The listing builds one solid part. Answer for the finished solid, in the listing's coordinates (mm). A direction names the side the tool comes from. Give positions to 0.01 mm unless a question says otherwise; leave off trailing zeros. Order: outer loops, then holes, each group sorted by start corner. A loop starts at its lowest first (then second) coordinate and runs counter-clockwise, first axis right, second up.
```python
from build123d import *

# Parameters (mm, degrees)
SKETCH1_R           = 1.8415
BOSS_EXTRUDE1_DEPTH = 3.81
CUT_EXTRUDE2_DEPTH  = 3.81
SKETCH2_R           = 3.4925
BOSS_EXTRUDE2_DEPTH = 31.75
SKETCH4_R           = 5.001975
SKETCH4_R_2         = 1.8415
SKETCH4_R_3         = 5.08
BOSS_EXTRUDE3_DEPTH = 6.35
SKETCH6_R           = 1.778
CUT_EXTRUDE3_DEPTH  = 5.08


with BuildPart() as part:
    # Sketch1 → Boss-Extrude1 (new body)
    with BuildSketch(Plane(origin=(0, 0, 0), x_dir=(1, 0, 0), z_dir=(0, 1, 0))):
        with BuildLine():
            Line((35.013825, 0), (38.50005, -3.486225))
            Line((38.50005, -3.486225), (41.802802741, -3.486225))
            ThreePointArc((41.802802741, -3.486225), (50.162319809, -2.012011059), (45.49775, 5.08))
            Line((45.49775, 5.08), (38.50005, 5.08))
            Line((38.50005, 5.08), (38.50005, 29.9974))
            Line((38.50005, 29.9974), (8.48995, 29.9974))
            Line((8.48995, 29.9974), (8.48995, 34.7599))
            ThreePointArc((8.48995, 34.7599), (3.40995, 39.8399), (-1.67005, 34.7599))
            Line((-1.67005, 34.7599), (-1.67005, 29.9974))
            Line((-1.67005, 29.9974), (-38.50005, 29.9974))
            Line((-38.50005, 29.9974), (-38.50005, 5.001975))
            ThreePointArc((-38.50005, 5.001975), (-42.036980442, -3.536930442), (-33.498075, 0))
            Line((-33.498075, 0), (35.013825, 0))
        make_face()
        with Locations((3.40995, 34.7599)):
            Circle(SKETCH1_R, mode=Mode.SUBTRACT)
        with Locations((45.49775, 0)):
            Circle(SKETCH1_R, mode=Mode.SUBTRACT)
        with Locations((-38.50005, 0)):
            Circle(SKETCH1_R, mode=Mode.SUBTRACT)
    extrude(amount=BOSS_EXTRUDE1_DEPTH)

    # Sketch3 → Cut-Extrude2 (cut)
    with BuildSketch(Plane(origin=(0, 0, 0), x_dir=(1, 0, 0), z_dir=(0, 1, 0))):
        with BuildLine():
            Line((-38.50005, 8.176975), (-38.50005, 29.9974))
            Line((-38.50005, 29.9974), (-4.84505, 29.9974))
            ThreePointArc((-4.84505, 29.9974), (-17.79061216, 13.099833084), (-38.50005, 8.176975))
        make_face()
    extrude(amount=CUT_EXTRUDE2_DEPTH, mode=Mode.SUBTRACT)

    # Sketch2 → Boss-Extrude2 (add)
    with BuildSketch(Plane(origin=(0, 0, 0), x_dir=(1, 0, 0), z_dir=(0, 1, 0))):
        with Locations((-15.55115, 14.9963886)):
            Circle(SKETCH2_R)
        with Locations((22.54885, 14.9963886)):
            Circle(SKETCH2_R)
    extrude(amount=BOSS_EXTRUDE2_DEPTH)

    # Sketch4 → Boss-Extrude3 (add)
    with BuildSketch(Plane.XZ):
        with Locations((-38.50005, 0)):
            Circle(SKETCH4_R)
        with Locations((-38.50005, 0)):
            Circle(SKETCH4_R_2, mode=Mode.SUBTRACT)
        with Locations((45.49775, 0)):
            Circle(SKETCH4_R_3)
        with Locations((45.49775, 0)):
            Circle(SKETCH4_R_2, mode=Mode.SUBTRACT)
        with Locations((3.40995, -34.7599)):
            Circle(SKETCH4_R_3)
        with Locations((3.40995, -34.7599)):
            Circle(SKETCH4_R_2, mode=Mode.SUBTRACT)
    extrude(amount=BOSS_EXTRUDE3_DEPTH)

    # Sketch6 → Cut-Extrude3 (cut)
    with BuildSketch(Plane(origin=(0, 31.75, 0), x_dir=(1, 0, 0), z_dir=(0, 1, 0))):
        with Locations((-15.55115, 14.9963886)):
            Circle(SKETCH6_R)
    extrude(amount=-CUT_EXTRUDE3_DEPTH, mode=Mode.SUBTRACT)


solid = part.part
```
1) For a pull along X with two mould halves and no side action, classify faces 4 (the cylindrical face through (-18.125, 15.653, -17.357)), 5 (the cylindrical face through (2.31, -2.33, -39.72)), 6 (the flat face through (38.5, 2, -17)), 7 (the cylindrical face through (-40.34, -1.2, 0.08)) as +X half, -X half, draft (parallel to the pull), parting line (faces both ways), or undercut.
Geometry says:
face 4: undercut
face 5: parting line
face 6: +X half
face 7: undercut
2) Given P1, Ø3, axis at x = 42, y = 1.5, coming from the -Z side; P2, Ø6, axis at x = 25, y = 5.5, coming from the +Z side; P3, Ø8, axis at x = -14, y = 22.5, coming from the -Z side; P4, Ø3.5, axis at x = 45.5, z = 0, coming from the +Y side, each flat-ended and moving along its own axis, determine where each tip first touches the part or whether it passes through.
Geometry says:
P1: stops at z = -5.08
P2: stops at z = 0
P3: stops at z = -18.49
P4: passes through
3) Find section D-D (x = 14). Write down the section's boundary in (y, z), then the cut area to 3 significant figures.
Geometry says:
outline: (0, -30) - (3.81, -30) - (3.81, 0) - (0, 0) - close
area: 114 mm2
4) Find section B-B (x = 4). Write down the section's boundary in (y, z), then the cut area to 3 significant figures.
Geometry says:
outline: (-6.35, -39.81) - (3.81, -39.81) - (3.81, -36.5) - (-6.35, -36.5) - close; (-6.35, -33.02) - (3.81, -33.02) - (3.81, 0) - (0, 0) - (0, -29.71) - (-6.35, -29.71) - close
area: 180 mm2
5) Find section A-A (y = 2.5). Count the separate pieces of the cut face and the enclosed holes in it, then the cut area to 3 significant figures.
Geometry says:
separate pieces: 1
enclosed holes: 3
area: 1,990 mm2
6) Find section C-C (y = 21). Write down the section's boundary in (x, z) (1 decimal).
Geometry says:
outline: circle Ø7 at (-15.6, -15); circle Ø7 at (22.5, -15)
7) A tool of negligible diameter and unlimited length cuts with its end or side. For faces 1 (the flat face through (40, 2, 3.486)), 2 (the flat face through (24, 2, -29.997)), 3 (the cylindrical face through (19.06, 17.58, -15.15)), from which of +Z, -Z, +X, -X, +Y, -Y can it reach the whole face along a straight path? Write none if from no direction.
Geometry says:
face 1: +Z, +Y, -Y
face 2: -Z, +X, +Y, -Y
face 3: +Y
8) Straight lines are drawn through the part: probe 1 along X at (y, z) = (-1, 0); probe 2 along Y at (x, z) = (26, -5.5); probe 3 along Z at (x, y) = (24, 2.5). For each, find the intervals that lie inside material, in ascending order.
Geometry says:
probe 1: x = -43.5 to -40.34, -36.66 to -33.5, 40.42 to 43.66, 47.34 to 50.58
probe 2: y = 0 to 3.81
probe 3: z = -30 to 0
